The listing builds one solid part. Answer for the finished solid, in the listing's coordinates (mm). A direction names the side the tool comes from. Round coordinates to 2 decimals unless told otherwise and drop trailing zeros. Loops run counter-clockwise (first coordinate to the right, second up) from the corner with the lowest first, then second, coordinate; pieces in that order, holes last. Notation, with made-up numbers: M 9.25,59 L 29.25,59 A22 ccw 29.25,96 Z; hole C 41,81.25 d1. An arc over 180 degrees is marked long. Answer as a JSON object with one key per item and string values.
```python
from build123d import *

# Parameters (mm, degrees)
SKETCH007_R     = 3.0625
PAD002_DEPTH    = 22.5
POCKET005_DEPTH = 22.5
POCKET006_DEPTH = 22.5
SKETCH010_R     = 3.875
POCKET007_DEPTH = 10
SKETCH011_W     = 2.5
SKETCH011_H     = 12.25
POCKET008_DEPTH = 15
SKETCH012_W     = 2.5
SKETCH012_H     = 9.3
POCKET009_DEPTH = 9.25
SKETCH013_W     = 2.5
SKETCH013_H     = 12.25
POCKET010_DEPTH = 15
SKETCH014_W     = 2.5
SKETCH014_H     = 9.8
POCKET011_DEPTH = 9.25
SKETCH031_R     = 1.6
POCKET019_DEPTH = 5
POCKET020_DEPTH = 2


with BuildPart() as part:
    # Sketch007 → Pad002 (new body)
    with BuildSketch(Plane.XZ):
        Polygon((-56, -7), (56, -7), (56, 2), (75, 2), (75, 7), (-75, 7), (-75, 2), (-56, 2), align=None)
        with Locations((-14, 0)):
            Circle(SKETCH007_R, mode=Mode.SUBTRACT)
        with Locations((14, 0)):
            Circle(SKETCH007_R, mode=Mode.SUBTRACT)
        with Locations((-26, 0)):
            Circle(SKETCH007_R, mode=Mode.SUBTRACT)
        with Locations((26, 0)):
            Circle(SKETCH007_R, mode=Mode.SUBTRACT)
    extrude(amount=PAD002_DEPTH)

    # Sketch008 (on Face3 of Pad002) → Pocket005 (cut)
    with BuildSketch(Plane(origin=(-56, 0, 0), x_dir=(0, 0, -1), z_dir=(-1, 0, 0))):
        Polygon((5, 22.5), (3, 22.5), (5, 0), (12, 0), (12, 22.5), align=None)
    extrude(amount=-POCKET005_DEPTH, mode=Mode.SUBTRACT)

    # Sketch009 (on Face11 of Pocket005) → Pocket006 (cut)
    with BuildSketch(Plane(origin=(56, 0, 0), x_dir=(0, 0, 1), z_dir=(1, 0, 0))):
        Polygon((-4.9, 0), (-11.9, 0), (-11.9, 22.5), (-4.9, 22.5), (-2.9, 22.5), align=None)
    extrude(amount=-POCKET006_DEPTH, mode=Mode.SUBTRACT)

    # Sketch010 (on Face8 of Pocket006) → Pocket007 (cut)
    with BuildSketch(Plane(origin=(0, -0.4409603136, -4.9608035277), x_dir=(1, 0, 0), z_dir=(0, -0.0885397903, -0.9960726407))):
        with Locations((-44.75, 11.3)):
            Circle(SKETCH010_R)
        with Locations((44.75, 11.3)):
            Circle(SKETCH010_R)
    extrude(amount=-POCKET007_DEPTH, mode=Mode.SUBTRACT)

    # Sketch011 (on Face13 of Pocket007) → Pocket008 (cut)
    with BuildSketch(Plane(origin=(56, 0, 0), x_dir=(0, 0, 1), z_dir=(1, 0, 0))):
        with Locations((0.75, 6.125)):
            Rectangle(SKETCH011_W, SKETCH011_H)
    extrude(amount=-POCKET008_DEPTH, mode=Mode.SUBTRACT)

    # Sketch012 (on Face15 of Pocket008) → Pocket009 (cut)
    with BuildSketch(Plane(origin=(41, 0, 0), x_dir=(0, 0, 1), z_dir=(1, 0, 0))):
        with Locations((0.75, 7.6)):
            Rectangle(SKETCH012_W, SKETCH012_H)
    extrude(amount=-POCKET009_DEPTH, mode=Mode.SUBTRACT)

    # Sketch013 (on Face7 of Pocket009) → Pocket010 (cut)
    with BuildSketch(Plane(origin=(-56, 0, 0), x_dir=(0, 0, -1), z_dir=(-1, 0, 0))):
        with Locations((-0.75, 6.125)):
            Rectangle(SKETCH013_W, SKETCH013_H)
    extrude(amount=-POCKET010_DEPTH, mode=Mode.SUBTRACT)

    # Sketch014 (on Face9 of Pocket010) → Pocket011 (cut)
    with BuildSketch(Plane(origin=(-41, 0, 0), x_dir=(0, 0, -1), z_dir=(-1, 0, 0))):
        with Locations((-0.75, 7.35)):
            Rectangle(SKETCH014_W, SKETCH014_H)
    extrude(amount=-POCKET011_DEPTH, mode=Mode.SUBTRACT)

    # Sketch031 (on Face2 of Pocket011) → Pocket019 (cut)
    with BuildSketch(Plane(origin=(0, 0, 7), x_dir=(-1, 0, 0), z_dir=(0, 0, 1))):
        with Locations((-66.75, 11.25)):
            Circle(SKETCH031_R)
        with Locations((66.75, 11.25)):
            Circle(SKETCH031_R)
    extrude(amount=-POCKET019_DEPTH, mode=Mode.SUBTRACT)

    # Sketch032 (on Face22 of Pocket019) → Pocket020 (cut)
    with BuildSketch(Plane(origin=(0, 0, 2), x_dir=(1, 0, 0), z_dir=(0, 0, -1))):
        Polygon((-65.125, 8.4354174377), (-63.5, 11.25), (-65.125, 14.0645825623), (-68.375, 14.0645825623), (-70, 11.25), (-68.375, 8.4354174377), align=None)
        Polygon((68.375, 8.4354174377), (70, 11.25), (68.375, 14.0645825623), (65.125, 14.0645825623), (63.5, 11.25), (65.125, 8.4354174377), align=None)
    extrude(amount=-POCKET020_DEPTH, mode=Mode.SUBTRACT)


solid = part.part
```
Item 1: Determine the mould class of faces 1 (the face through (-65, -13, 4)), 2 (the face through (75, -11, 4)), 3 (the face through (-68.276, -11.731, 5.521)), 4 (the face through (1, -11, 7)) for opening direction X: released by +X, released by -X, zero draft, split by the parting line, or undercut.
Values follow:
{"face 1": "undercut", "face 2": "released by +X", "face 3": "undercut", "face 4": "zero draft"}
Item 2: Flat-ended cylindrical pins translate along their axes: P1, Ø10, axis at x = -39, y = -15.5, coming from the -Z side; P2, Ø1.2, axis at y = -10, z = -4.5, coming from the -X side; P3, Ø1, axis at x = 6.5, z = 0.5, coming from the +Y side; P4, Ø0.7, axis at y = -1, z = 1, coming from the -X side. Find the tip coordinate at first contact, or state that the pin passes through.
Values follow:
{"P1": "z = -4.07", "P2": "x = -56", "P3": "y = 0", "P4": "x = -41"}
Item 3: Straight lines are drawn through the part: line 1 (X direction, y = -11.25, z = 5.45); line 2 (Z direction, x = 26, y = -15.5); line 3 (X direction, y = -15.5, z = -1.5). For each, find the intervals that lie inside material, in ascending order.
Values follow:
{"line 1": "-75 to -68.35, -65.15 to -48.61, -40.89 to 40.89, 48.61 to 65.15, 68.35 to 75", "line 2": "-7 to -3.06, 3.06 to 7", "line 3": "-56 to -28.67, -23.33 to -16.67, -11.33 to 11.33, 16.67 to 23.33, 28.67 to 56"}
Item 4: Which of the six approach directions +Z, -Z, +X, -X, +Y, -Y give full straight-line access (tool end or side, diameter ignored) to faces 5 (the face through (-41, -1, 1)), 6 (the face through (-44.804, -10.865, 6.005)), 7 (the face through (-33.5, -11, -5)), 8 (the face through (41, -1, 1))?
Values follow:
{"face 5": "-X, +Y", "face 6": "none", "face 7": "-Z, -X, -Y", "face 8": "+X, +Y"}
Item 5: The part is cut by section B-B (y = -19.75). Give the vertices of the cut face in (x, z) (1 decimal), then the cut area to 3 significant figures.
Values follow:
{"outline": "M -75,2 L -56,2 L -56,-3.2 L -33.5,-3.2 L -33.5,-7 L 33.5,-7 L 33.5,-3.1 L 56,-3.1 L 56,2 L 75,2 L 75,7 L -75,7 Z; hole C -26,0 d6.1; hole C -14,0 d6.1; hole C 14,0 d6.1; hole C 26,0 d6.1", "area": "1,470 mm^2"}
Item 6: The part is cut by section C-C (x = -26). Give the vertices of the cut face in (y, z).
Values follow:
{"outline": "M -22.5,-7 L 0,-7 L 0,-3.06 L -22.5,-3.06 Z; M -22.5,3.06 L 0,3.06 L 0,7 L -22.5,7 Z"}
Item 7: The part is cut by section A-A (x = 66.75). Give the vertices of the cut face in (y, z).
Values follow:
{"outline": "M -22.5,2 L -14.06,2 L -14.06,4 L -12.85,4 L -12.85,7 L -22.5,7 Z; M -9.65,4 L -8.44,4 L -8.44,2 L 0,2 L 0,7 L -9.65,7 Z"}
